Autodesk Inventor part; units mm, degrees
ref_plane "Plano de trabajo1" through (0, -46.2161, 0) normal (0, 0, 1) x (-1, 0, 0)
ref_plane "YZ Plane" through (0, 0, 0) normal (1, 0, 0) x (0, 1, 0)
ref_plane "XZ Plane" through (0, 0, 0) normal (0, 1, 0) x (-1, 0, 0)
ref_plane "Plano de trabajo1" through (0, -46.2161, 0) normal (0, 0, 1) x (-1, 0, 0)
sketch "Boceto1" plane through (0, -46.2161, 0) normal (0, 0, 1) x (-1, 0, 0)
  line L0 (14.8515, 14.9812) -> (54.8515, 14.9812)
  line L1 (14.8515, -15) -> (14.8515, 14.9812)
  line L2 (54.8515, -15) -> (14.8515, -15)
  line L3 (54.8515, 14.9812) -> (54.8515, -15)
  circle A0 centre (19.3515, 11) radius 1.25
  circle A1 centre (19.3515, -11.0188) radius 1.25
  point P0 (0, -46.2161)
extrude "Extrusión1" add sketch "Boceto1" against normal blind 5
sketch "Boceto2" plane through (0, -46.2161, -5) normal (0, 0, -1) x (-1, 0, 0)
  line L0 (54.8515, -14.9812) -> (54.8515, 15)
  line L1 (54.8515, 15) -> (14.8515, 15)
  line L2 (54.8515, -14.9812) -> (49.8515, -14.9812)
  line L3 (49.8515, -14.9812) -> (49.8515, 15)
  line L4 (49.8515, 15) -> (54.8515, 15)
  line L5 (54.8515, 15) -> (54.8515, -14.9812)
  point P0 (0, 46.2161)
  dimension "d2" = 5
extrude "Extrusión2" add sketch "Boceto2" along normal blind 35
sketch "Boceto3" plane through (-49.8515, -61.1974, -5) normal (1, 0, 0) x (0, 0, -1)
  line L0 (0, 0) -> (35, 0)
  line L1 (35, 0) -> (35, 29.9812)
  line L2 (35, 29.9812) -> (0, 29.9812)
  line L3 (0, 29.9812) -> (0, 0)
  line L4 (0, 0) -> (35, 0)
  line L5 (0, 29.9812) -> (35, 29.9812)
  circle A0 centre (17.5, 14.9906) radius 5.5
  point P0 (-5, 61.1974)
  dimension "d5" = 11
extrude "Extrusión3" cut sketch "Boceto3" against normal blind 35 contours A0
thread "Rosca1"
properties part number "Soporte"
The model under review builds one solid part; all positions refer to its coordinate system, in mm. A direction names the side the tool comes from. Round coordinates to 2 decimals unless told otherwise and drop trailing zeros. Write each loop counter-clockwise with the first axis right and the second up, starting at its lowest first coordinate (ties: lowest second). Pieces come first, ordered by that corner, then holes. Notation, with made-up numbers: (70, 51) -> (118, 51) arc R27 cw to (118, 81) -> close; hole circle Ø5 at (29.25, 83.5). An arc over 180 degrees is marked (long way). Answer as a JSON object with one key per item and string values.
1. Clearance check with flat-ended pins moving along their axes: pin 1 (8 mm diameter, centred on x = -45.5, y = -36, fed in from -Z); pin 2 (2 mm diameter, centred on x = -19.35, y = -35.2, fed in from +Z); pin 3 (1 mm diameter, centred on y = -51, z = -31, fed in from +X). State where each tip first meets the part, or that it passes through.
Results found:
{"pin 1": "stops at z = -5", "pin 2": "passes through", "pin 3": "stops at x = -49.85"}
2. Machinability: for faces 5 (the face through (-54.852, -46, -15)), 6 (the face through (-49.852, -53, -22)), which of the approach directions +Z, -Z, +X, -X, +Y, -Y give a long, thin tool a straight path to every point of the face, cutting with its end or side? Answer none if there is none.
Results found:
{"face 5": "+Z, -Z, -X, +Y, -Y", "face 6": "-Z, +X, +Y, -Y"}
3. We need section D-D on y = -53. State the section outline as (x, z) points, and give its area (3 significant figures).
Results found:
{"outline": "(-54.85, -40) -> (-49.85, -40) -> (-49.85, -5) -> (-14.85, -5) -> (-14.85, 0) -> (-54.85, 0) -> close", "area": "375 mm^2"}
4. We need section A-A on z = -22.5. State the section outline as (x, y) points.
Results found:
{"outline": "(-54.85, -61.2) -> (-49.85, -61.2) -> (-49.85, -51.71) -> (-54.85, -51.71) -> close; (-54.85, -40.71) -> (-49.85, -40.71) -> (-49.85, -31.22) -> (-54.85, -31.22) -> close"}
5. We need section C-C on x = -51. State the section outline as (y, z) points.
Results found:
{"outline": "(-61.2, -40) -> (-31.22, -40) -> (-31.22, 0) -> (-61.2, 0) -> close; hole circle Ø11 at (-46.21, -22.5)"}
6. The part is to be moulded in two halves that separate along X. For faces 1 (the face through (-19.081, -33.977, -2.465)), 2 (the face through (-35, -46, 0)), 3 (the face through (-14.852, -46, -2)), 4 (the face through (-19.93, -56.11, -2.46)), say which applies: pulls with the +X half, pulls with the -X half, needs draft (parallel to the pull), parting line crosses it, or undercut.
Results found:
{"face 1": "undercut", "face 2": "needs draft", "face 3": "pulls with the +X half", "face 4": "undercut"}
7. We need section B-B on y = -50. State the section outline as (x, z) points, and give its area (3 significant figures).
Results found:
{"outline": "(-54.85, -40) -> (-49.85, -40) -> (-49.85, -26.48) -> (-54.85, -26.48) -> close; (-54.85, -18.52) -> (-49.85, -18.52) -> (-49.85, -5) -> (-14.85, -5) -> (-14.85, 0) -> (-54.85, 0) -> close", "area": "335 mm^2"}
8. To check wall thickness, follow line 1 along X through (y, z) = (-37.25, -8); line 2 along Y through (x, z) = (-51.4, -22.5); line 3 along Z through (x, y) = (-44, -40.25). State the ranges of each line that lie inside material, in increasing order.
Results found:
{"line 1": "x = -54.85 to -49.85", "line 2": "y = -61.2 to -51.71, -40.71 to -31.22", "line 3": "z = -5 to 0"}
